```python
from build123d import *

# Parameters (mm, degrees)
SKETCH1_W           = 15
SKETCH1_H           = 30
BOSS_EXTRUDE1_DEPTH = 2
SKETCH2_W           = 2
SKETCH2_H           = 30
BOSS_EXTRUDE2_DEPTH = 53
SKETCH3_R           = 15
SKETCH3_R_2         = 12.5
BOSS_EXTRUDE3_DEPTH = 92
BOSS_EXTRUDE4_START = -2
SKETCH4_R           = 12.5
SKETCH4_R_2         = 11.5
BOSS_EXTRUDE4_DEPTH = 2
SKETCH7_R           = 3
CUT_EXTRUDE1_DEPTH  = 10


with BuildPart() as part:
    # Sketch1 → Boss-Extrude1 (new body)
    with BuildSketch(Plane(origin=(0, 0, 0), x_dir=(1, 0, 0), z_dir=(0, 1, 0))):
        Rectangle(SKETCH1_W, SKETCH1_H)
    extrude(amount=BOSS_EXTRUDE1_DEPTH)

    # Sketch2 → Boss-Extrude2 (add)
    with BuildSketch(Plane(origin=(0, 2, 0), x_dir=(1, 0, 0), z_dir=(0, 1, 0))):
        with Locations((-6.5, 0)):
            Rectangle(SKETCH2_W, SKETCH2_H)
    extrude(amount=BOSS_EXTRUDE2_DEPTH)

    # Sketch3 → Boss-Extrude3 (add)
    with BuildSketch(Plane(origin=(-5.5, 0, 0), x_dir=(0, 0, -1), z_dir=(1, 0, 0))):
        with Locations((0, 40)):
            Circle(SKETCH3_R)
        with Locations((0, 40)):
            Circle(SKETCH3_R_2, mode=Mode.SUBTRACT)
    extrude(amount=BOSS_EXTRUDE3_DEPTH)

    # Sketch4 → Boss-Extrude4 (add)
    with BuildSketch(Plane(origin=(86.5, 0, 0), x_dir=(0, 0, -1), z_dir=(1, 0, 0)).offset(BOSS_EXTRUDE4_START)):
        with Locations((0, 40)):
            Circle(SKETCH4_R)
        with Locations((0, 40)):
            Circle(SKETCH4_R_2, mode=Mode.SUBTRACT)
    extrude(amount=BOSS_EXTRUDE4_DEPTH)

    # Sketch7 → Cut-Extrude1 (cut)
    with BuildSketch(Plane(origin=(0, 2, 0), x_dir=(1, 0, 0), z_dir=(0, 1, 0))):
        with Locations(Location((1, -9, 0), (0, 0, 270))):
            Circle(SKETCH7_R)
        with Locations(Location((1, 9, 0), (0, 0, 270))):
            Circle(SKETCH7_R)
    extrude(amount=-CUT_EXTRUDE1_DEPTH, mode=Mode.SUBTRACT)


solid = part.part
```
The listing builds one solid part. Answer for the finished solid, in the listing's coordinates (mm). A direction names the side the tool comes from. Round coordinates to 2 decimals unless told otherwise and drop trailing zeros. Loops run counter-clockwise (first coordinate to the right, second up) from the corner with the lowest first, then second, coordinate; pieces in that order, holes last. Notation, with made-up numbers: (85, -28) - (141, -28) arc R18 cw to (141, -17) - close; hole circle Ø6 at (-28, 83.5). An arc over 180 degrees is marked (long way). Return JSON: item names as keys, results as strings. Group by question number.
1. The part is cut by section B-B on z = -9. Determine the outline of the cut face in (x, y).
2. The part is cut by section A-A on x = 1. Determine the outline of the cut face in (y, z), then the cut area to 3 significant figures.
3. The mould has two halves that part along Z. Classify faces 1 (the flat face through (7.5, 1, 0)), 2 (the cylindrical face through (85.486, 28.773, 2.493)), 3 (the flat face through (-6, 23, -15)): pulls with the +Z half, pulls with the -Z half, needs draft (parallel to the pull), parting line crosses it, or undercut.
4. Consider probe 1 along X at (y, z) = (0.75, 9); probe 2 along Y at (x, z) = (-2, 5.25); probe 3 along Y at (x, z) = (-2.5, 4). Determine where each line is inside the solid, lowest interval first.
5. Which of the six approach directions +Z, -Z, +X, -X, +Y, -Y give full straight-line access (tool end or side, diameter ignored) to faces 4 (the flat face through (-5.5, 52, -12)), 5 (the flat face through (-5.5, 40, 0)), 6 (the cylindrical face through (39.856, 54.872, 1.953)), 7 (the flat face through (-5.5, 51, 12))?
6. The part is cut by section C-C on y = 43.5. Determine the outline of the cut face in (x, z).
7. Each of these flat-tipped pins is pushed along its axis until it touches: P1, Ø1, axis at y = 1.5, z = -0.5, coming from the +X side; P2, Ø1.5, axis at x = 52.5, z = -1.5, coming from the +Y side; P3, Ø2, axis at x = 25, y = 34, coming from the -Z side. Where does it stop, or does it pass through?
8. The part is cut by section D-D on x = 10.5. Determine the outline of the cut face in (y, z).
Resolved:
{
 "1": {"outline": "(-7.5, 0) - (-2, 0) - (-2, 2) - (-5.5, 2) - (-5.5, 28) - (86.5, 28) - (86.5, 32.84) - (84.5, 32.84) - (84.5, 31.33) - (-5.5, 31.33) - (-5.5, 48.67) - (84.5, 48.67) - (84.5, 47.16) - (86.5, 47.16) - (86.5, 52) - (-5.5, 52) - (-5.5, 55) - (-7.5, 55) - close; (4, 0) - (7.5, 0) - (7.5, 2) - (4, 2) - close"},
 "2": {"outline": "(0, -15) - (2, -15) - (2, -12) - (0, -12) - close; (0, -6) - (2, -6) - (2, 6) - (0, 6) - close; (0, 12) - (2, 12) - (2, 15) - (0, 15) - close; circle Ø30 at (40, 0); hole circle Ø25 at (40, 0)", "area": "252 mm²"},
 "3": {"face 1": "needs draft", "face 2": "undercut", "face 3": "pulls with the -Z half"},
 "4": {"probe 1": "x = -7.5 to -2, 4 to 7.5", "probe 2": "y = 0 to 2, 25.95 to 28.66, 51.34 to 54.05", "probe 3": "y = 0 to 2, 25.54 to 28.16, 51.84 to 54.46"},
 "5": {"face 4": "-Z, +X, +Y", "face 5": "none", "face 6": "+X", "face 7": "+Z, +X, +Y"},
 "6": {"outline": "(-7.5, -15) - (-5.5, -15) - (-5.5, -14.59) - (86.5, -14.59) - (86.5, -10.95) - (84.5, -10.95) - (84.5, -12) - (-5.5, -12) - (-5.5, 12) - (84.5, 12) - (84.5, 10.95) - (86.5, 10.95) - (86.5, 14.59) - (-5.5, 14.59) - (-5.5, 15) - (-7.5, 15) - close"},
 "7": {"P1": "stops at x = 7.5", "P2": "stops at y = 54.98", "P3": "stops at z = -14.14"},
 "8": {"outline": "circle Ø30 at (40, 0); hole circle Ø25 at (40, 0)"}
}
